CAD build for the part. Positions are in the model's coordinates, mm. A direction names the side the tool comes from. Give positions to 0.01 mm unless a question says otherwise; leave off trailing zeros. Order: outer loops, then holes, each group sorted by start corner. A loop starts at its lowest first (then second) coordinate and runs counter-clockwise, first axis right, second up.
Item 1: Wall check: L1, parallel to Y at x = -12.5, z = 89.5; L2, parallel to Y at x = -3, z = 74. Give the ranges that are in metal, low to high.
Item 2: Which spindle directions (+Z, -Z, +X, -X, +Y, -Y) get a long thin tool onto all of the face, cutting with end or side? Do faces 4 (the flat face through (-20, -10, 49)), 5 (the flat face through (-8, 3, 49)). Say none if no direction does.
Item 3: Flat gauge pins, fed straight in: P1, Ø3, axis at y = 7.5, z = 26.5, coming from the +X side; P2, Ø8, axis at y = 11.5, z = 58, coming from the +X side; P3, Ø6, axis at y = -2.5, z = 61, coming from the +X side. Where does each tip first touch, or does it go through?
Item 4: Band-saw the part on B-B on z = 79. Count the separate pieces of the cut face and the enclosed holes in it, plus the area to 3 significant figures.
Item 5: Band-saw the part on A-A on x = -13. Give the cut face in (y, z), plus the area to 3 significant figures.
Item 6: Two-plate mould, pull along X, no slides. Class faces 1 (the flat face through (5.295, 5.701, 49.3)), 2 (the flat face through (5, -15.5, 49)), 3 (the flat face through (-3, -4, 100)): released by +X, released by -X, zero draft, split by the parting line, or undercut.
```python
from build123d import *

# Parameters (mm, degrees)
EXTRUDE_1_DEPTH = 100


with BuildPart() as part:
    # 草图1 → 凸台-拉伸1 (new body)
    with BuildSketch(Plane.XY):
        with BuildLine():
            Line((-20, -15.5), (-20, -5.2))
            Line((-20, -5.2), (-19, -5.2))
            Line((-19, -5.2), (-19, -4.2))
            Line((-19, -4.2), (-15.5, -4.2))
            Line((-15.5, -4.2), (-15.5, -6.3))
            Line((-15.5, -6.3), (-18, -6.3))
            Line((-18, -6.3), (-18, -10.05))
            ThreePointArc((-18, -10.05), (-17.941421356, -10.191421356), (-17.8, -10.25))
            Line((-17.8, -10.25), (-11.876345597, -10.25))
            Line((-11.876345597, -10.25), (-8, -6.373654403))
            Line((-8, -6.373654403), (-8, -0.5))
            Line((-8, -0.5), (-7.5, 0))
            Line((-7.5, 0), (-8, 0.5))
            Line((-8, 0.5), (-8, 6.373654403))
            Line((-8, 6.373654403), (-11.876345597, 10.25))
            Line((-11.876345597, 10.25), (-17.8, 10.25))
            ThreePointArc((-17.8, 10.25), (-17.941421356, 10.191421356), (-18, 10.05))
            Line((-18, 10.05), (-18, 6.3))
            Line((-18, 6.3), (-15.5, 6.3))
            Line((-15.5, 6.3), (-15.5, 4.2))
            Line((-15.5, 4.2), (-19, 4.2))
            Line((-19, 4.2), (-19, 5.2))
            Line((-19, 5.2), (-20, 5.2))
            Line((-20, 5.2), (-20, 15.5))
            ThreePointArc((-20, 15.5), (-18.681980515, 18.681980515), (-15.5, 20))
            Line((-15.5, 20), (-9.004415588, 20))
            Line((-9.004415588, 20), (20, -9.004415588))
            Line((20, -9.004415588), (20, -15.5))
            ThreePointArc((20, -15.5), (18.681980515, -18.681980515), (15.5, -20))
            Line((15.5, -20), (5.2, -20))
            Line((5.2, -20), (5.2, -19))
            Line((5.2, -19), (4.2, -19))
            Line((4.2, -19), (4.2, -15.5))
            Line((4.2, -15.5), (6.3, -15.5))
            Line((6.3, -15.5), (6.3, -18))
            Line((6.3, -18), (10.05, -18))
            ThreePointArc((10.05, -18), (10.191421356, -17.941421356), (10.25, -17.8))
            Line((10.25, -17.8), (10.25, -11.876345597))
            Line((10.25, -11.876345597), (6.373654403, -8))
            Line((6.373654403, -8), (0.5, -8))
            Line((0.5, -8), (0, -7.5))
            Line((0, -7.5), (-0.5, -8))
            Line((-0.5, -8), (-6.373654403, -8))
            Line((-6.373654403, -8), (-10.25, -11.876345597))
            Line((-10.25, -11.876345597), (-10.25, -17.8))
            ThreePointArc((-10.25, -17.8), (-10.191421356, -17.941421356), (-10.05, -18))
            Line((-10.05, -18), (-6.3, -18))
            Line((-6.3, -18), (-6.3, -15.5))
            Line((-6.3, -15.5), (-4.2, -15.5))
            Line((-4.2, -15.5), (-4.2, -19))
            Line((-4.2, -19), (-5.2, -19))
            Line((-5.2, -19), (-5.2, -20))
            Line((-5.2, -20), (-15.5, -20))
            ThreePointArc((-15.5, -20), (-18.681980515, -18.681980515), (-20, -15.5))
        make_face()
        with BuildLine():
            Line((-18.2, -15.5), (-18.2, -11.95))
            ThreePointArc((-18.2, -11.95), (-18.141421356, -11.808578644), (-18, -11.75))
            Line((-18, -11.75), (-11.95, -11.75))
            ThreePointArc((-11.95, -11.75), (-11.808578644, -11.808578644), (-11.75, -11.95))
            Line((-11.75, -11.95), (-11.75, -18))
            ThreePointArc((-11.75, -18), (-11.808578644, -18.141421356), (-11.95, -18.2))
            Line((-11.95, -18.2), (-15.5, -18.2))
            ThreePointArc((-15.5, -18.2), (-17.409188309, -17.409188309), (-18.2, -15.5))
        make_face(mode=Mode.SUBTRACT)
        with BuildLine():
            Line((-18.2, 15.5), (-18.2, 11.95))
            ThreePointArc((-18.2, 11.95), (-18.141421356, 11.808578644), (-18, 11.75))
            Line((-18, 11.75), (-11.95, 11.75))
            ThreePointArc((-11.95, 11.75), (-11.808578644, 11.808578644), (-11.75, 11.95))
            Line((-11.75, 11.95), (-11.75, 18))
            ThreePointArc((-11.75, 18), (-11.808578644, 18.141421356), (-11.95, 18.2))
            Line((-11.95, 18.2), (-15.5, 18.2))
            ThreePointArc((-15.5, 18.2), (-17.409188309, 17.409188309), (-18.2, 15.5))
        make_face(mode=Mode.SUBTRACT)
        with BuildLine():
            Line((-6.373654403, 8), (-10.25, 11.876345597))
            Line((-10.25, 11.876345597), (-10.25, 18.2))
            Line((-10.25, 18.2), (-9.75, 18.2))
            Line((-9.75, 18.2), (-0.403553391, 8.853553391))
            ThreePointArc((-0.403553391, 8.853553391), (-0.295167015, 8.308658284), (-0.757106781, 8))
            Line((-0.757106781, 8), (-6.373654403, 8))
        make_face(mode=Mode.SUBTRACT)
        with BuildLine():
            Line((8, -6.373654403), (11.876345597, -10.25))
            Line((11.876345597, -10.25), (18.2, -10.25))
            Line((18.2, -10.25), (18.2, -9.75))
            Line((18.2, -9.75), (8.853553391, -0.403553391))
            ThreePointArc((8.853553391, -0.403553391), (8.308658284, -0.295167015), (8, -0.757106781))
            Line((8, -0.757106781), (8, -6.373654403))
        make_face(mode=Mode.SUBTRACT)
        with BuildLine():
            Line((-3.181980515, -3.889087297), (-2.024471, -2.731577781))
            ThreePointArc((-2.024471, -2.731577781), (0, -3.4), (2.024471, -2.731577781))
            Line((2.024471, -2.731577781), (3.181980515, -3.889087297))
            ThreePointArc((3.181980515, -3.889087297), (3.889087297, -3.889087297), (3.889087297, -3.181980515))
            Line((3.889087297, -3.181980515), (2.731577781, -2.024471))
            ThreePointArc((2.731577781, -2.024471), (2.404163056, 2.404163056), (-2.024471, 2.731577781))
            Line((-2.024471, 2.731577781), (-3.181980515, 3.889087297))
            ThreePointArc((-3.181980515, 3.889087297), (-3.889087297, 3.889087297), (-3.889087297, 3.181980515))
            Line((-3.889087297, 3.181980515), (-2.731577781, 2.024471))
            ThreePointArc((-2.731577781, 2.024471), (-3.4, 0), (-2.731577781, -2.024471))
            Line((-2.731577781, -2.024471), (-3.889087297, -3.181980515))
            ThreePointArc((-3.889087297, -3.181980515), (-3.889087297, -3.889087297), (-3.181980515, -3.889087297))
        make_face(mode=Mode.SUBTRACT)
        with BuildLine():
            Line((15.5, -18.2), (11.95, -18.2))
            ThreePointArc((11.95, -18.2), (11.808578644, -18.141421356), (11.75, -18))
            Line((11.75, -18), (11.75, -11.95))
            ThreePointArc((11.75, -11.95), (11.808578644, -11.808578644), (11.95, -11.75))
            Line((11.95, -11.75), (18, -11.75))
            ThreePointArc((18, -11.75), (18.141421356, -11.808578644), (18.2, -11.95))
            Line((18.2, -11.95), (18.2, -15.5))
            ThreePointArc((18.2, -15.5), (17.409188309, -17.409188309), (15.5, -18.2))
        make_face(mode=Mode.SUBTRACT)
    extrude(amount=EXTRUDE_1_DEPTH)


solid = part.part
```
The answers:
1. L1: y = -20 to -18.2, -11.75 to -10.25, 10.25 to 11.75, 18.2 to 20
1. L2: y = -8 to -3.71, -2.29 to -1.6, 1.6 to 2.29, 3.71 to 8, 11.45 to 14
2. face 4: +Z, -Z, -X, +Y, -Y
2. face 5: +Z, -Z
3. P1: stops at x = 5
3. P2: stops at x = 3.5
3. P3: stops at x = 16.5
4. separate pieces: 1
4. enclosed holes: 6
4. area: 508 mm2
5. outline: (-20, 0) - (-18.2, 0) - (-18.2, 100) - (-20, 100) - close; (-11.75, 0) - (-10.25, 0) - (-10.25, 100) - (-11.75, 100) - close; (10.25, 0) - (11.75, 0) - (11.75, 100) - (10.25, 100) - close; (18.2, 0) - (20, 0) - (20, 100) - (18.2, 100) - close
5. area: 660 mm2
6. face 1: released by +X
6. face 2: undercut
6. face 3: zero draft
